Source: CAD feature listing. Evaluate the final solid. Frame: model axes, mm. Face numbers are marked on the shaded views. Coordinates: 2 decimals unless noted, no trailing zeros. Order: outer loops, then holes, each group sorted by start corner. A loop starts at its lowest first (then second) coordinate and runs counter-clockwise, first axis right, second up.
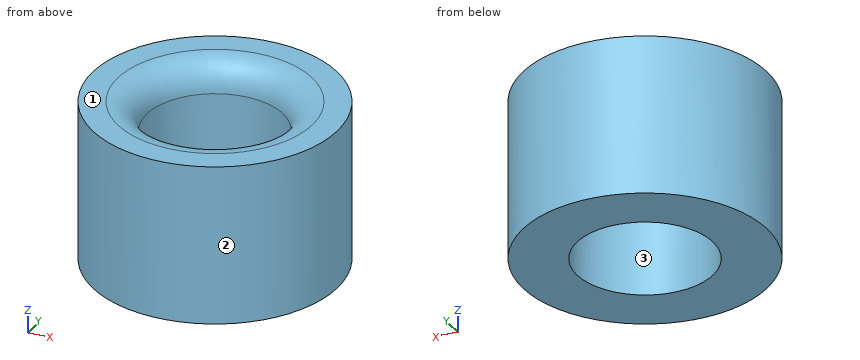
```python
from build123d import *

# Parameters (mm, degrees)
CYLINDER012_R     = 3.14
CYLINDER012_DEPTH = 4.1
CYLINDER013_R     = 1.75
CYLINDER013_DEPTH = 14
FILLET005_R       = 0.75


with BuildPart() as part:
    # Cylinder012 → Cylinder012 (join)
    with BuildSketch(Plane.XY.offset(12)):
        Circle(CYLINDER012_R)
    extrude(amount=CYLINDER012_DEPTH)

    # Cylinder013 → Cylinder013 (cut)
    with BuildSketch(Plane.XY.offset(3)):
        Circle(CYLINDER013_R)
    extrude(amount=CYLINDER013_DEPTH, mode=Mode.SUBTRACT)

    # Fillet005
    fillet005_edges = [part.edges().sort_by_distance(p)[0] for p in [
        (-1.75, 0, 16.1),
    ]]
    fillet(fillet005_edges, radius=FILLET005_R)


solid = part.part
```
Q1. Pin query (flat end, axial travel): P1, Ø1, axis at x = -1.5, z = 13, coming from the +Y side; P2, Ø1, axis at y = 2, z = 13.5, coming from the -X side. Return the tip coordinate at first contact, or that it passes through.
Solutions:
P1: stops at y = 2.98
P2: stops at x = -2.76
Q2. Material intervals for line 1 along Y through (x, z) = (0, 14.6); line 2 along X through (y, z) = (1.25, 13.7); line 3 along Y through (x, z) = (0.75, 12.75), sorted ascending.
Solutions:
line 1: y = -3.14 to -1.75, 1.75 to 3.14
line 2: x = -2.88 to -1.22, 1.22 to 2.88
line 3: y = -3.05 to -1.58, 1.58 to 3.05
Q3. Pull-direction query (X, two-part tool) for the marked faces 1, 2 and 3; classes: pulls with the +X half, pulls with the -X half, needs draft (parallel to the pull), parting line crosses it, or undercut.
Solutions:
face 1: needs draft
face 2: parting line crosses it
face 3: undercut
Q4. Section query A-A on x = 0. Output: boundary loops of the cut face in (y, z), plus the area to 3 significant figures.
Solutions:
outline: (-3.14, 12) - (-1.75, 12) - (-1.75, 15.35) arc R0.75 ccw to (-2.5, 16.1) - (-3.14, 16.1) - close; (1.75, 12) - (3.14, 12) - (3.14, 16.1) - (2.5, 16.1) arc R0.75 ccw to (1.75, 15.35) - close
area: 11.2 mm2
Q5. Section query D-D on z = 15.6. Output: boundary loops of the cut face in (x, y).
Solutions:
outline: circle Ø6.28 at (0, 0); hole circle Ø3.59 at (0, 0)
Q6. Section query C-C on z = 13.1. Output: boundary loops of the cut face in (x, y).
Solutions:
outline: circle Ø6.28 at (0, 0); hole circle Ø3.5 at (0, 0)
